Here's how the part is built. I have some questions about the finished solid (model axes, mm). A direction names the side the tool comes from. Give positions to 0.01 mm unless a question says otherwise; leave off trailing zeros. Loops run counter-clockwise (first coordinate to the right, second up) from the corner with the lowest first, then second, coordinate; pieces in that order, holes last. Notation, with made-up numbers: M 22,-19.5 L 64,-19.5 A18 cw 64,-13.5 Z; hole C 82.5,27.25 d9. An arc over 180 degrees is marked long. Answer as CSV lines item,"result". Start each with the question number.
Item 1: I want a section at A-A on y = 10. List the corners of the cut face in (x, z) for me, plus the area to 3 significant figures.
Item 2: If I drill on line 1 along Z through (x, y) = (-7.5, 10); line 2 along X through (y, z) = (11, 10); line 3 along Z through (x, y) = (2, 11), over which ranges is the centre line in solid material (lowest first)? Write a range as from..to.
Item 3: I want a section at B-B on z = 4.5. List the corners of the cut face in (x, y) for me.
Item 4: If we mould it in two halves opening along Y, with no side actions, what happens to faces 1 (the cylindrical face through (5.65, 3.52, -22.27)), 2 (the cylindrical face through (-7.062, 11.341, 8.694)), 3 (the flat face through (5.33, 2, 36.78)), 4 (the flat face through (-4, 0, 5))? For each: released by +Y, released by -Y, zero draft, split by the parting line, or undercut.
Item 5: I want a section at C-C on z = 34.5. List the corners of the cut face in (x, y) for me, plus the area to 3 significant figures.
Item 6: For faces 5 (the cylindrical face through (15.357, 11.341, 8.694)), 6 (the cylindrical face through (4.367, 3.521, 32.966)), 7 (the flat face through (-8.852, 10, 8)), 8 (the flat face through (17.148, 10, 8)), 9 (the cylindrical face through (4.214, 1.014, -28.538)), which set-ups out of +Z, -Z, +X, -X, +Y, -Y let a thin tool reach every point of the face, with its end or its side?
Item 7: I want a section at D-D on x = 32. List the corners of the cut face in (y, z) for me.
Item 8: Will these pins go through, and if not, where does the flat tip stop? P1, Ø8, axis at y = 12, z = 10.5, coming from the -X side; P2, Ø16, axis at x = 4.15, z = 5.46, coming from the +Y side; P3, Ø6, axis at x = -18, z = -15, coming from the +Y side; P4, Ø7, axis at y = 10, z = 5.46, coming from the +X side.
from build123d import *

# Parameters (mm, degrees)
SKETCH1_R           = 40
BOSS_EXTRUDE1_DEPTH = 5
SKETCH2_R           = 5
CUT_EXTRUDE1_DEPTH  = 15
SKETCH3_R           = 5
CUT_EXTRUDE2_DEPTH  = 3
SKETCH5_R           = 1.5
CUT_EXTRUDE3_DEPTH  = 33
BOSS_EXTRUDE2_START = 10
SKETCH6_R           = 10
SKETCH6_R_2         = 5
BOSS_EXTRUDE2_DEPTH = 10
SKETCH10_R          = 2.25
CUT_EXTRUDE4_DEPTH  = 45
BOSS_EXTRUDE3_START = 8
SKETCH11_R          = 3.5
SKETCH11_R_2        = 2.25
BOSS_EXTRUDE3_DEPTH = 8


with BuildPart() as part:
    # Sketch1 → Boss-Extrude1 (new body)
    with BuildSketch(Plane(origin=(0, 0, 0), x_dir=(1, 0, 0), z_dir=(0, 1, 0))):
        with Locations(Location((4.147627533, -5.460766911, 0), (0, 0, 270))):
            Circle(SKETCH1_R)
    extrude(amount=BOSS_EXTRUDE1_DEPTH)

    # Sketch2 → Cut-Extrude1 (cut)
    with BuildSketch(Plane(origin=(0, 5, 0), x_dir=(1, 0, 0), z_dir=(0, 1, 0))):
        with Locations(Location((4.147627533, -5.460766911, 0), (0, 0, 270))):
            Circle(SKETCH2_R)
    extrude(amount=-CUT_EXTRUDE1_DEPTH, mode=Mode.SUBTRACT)

    # Sketch3 → Cut-Extrude2 (cut)
    with BuildSketch(Plane(origin=(0, 5, 0), x_dir=(1, 0, 0), z_dir=(0, 1, 0))):
        with Locations(Location((4.147627533, 27.039233089, 0), (0, 0, 270))):
            Circle(SKETCH3_R)
        with Locations(Location((4.147627533, -37.960766911, 0), (0, 0, 270))):
            Circle(SKETCH3_R)
    extrude(amount=-CUT_EXTRUDE2_DEPTH, mode=Mode.SUBTRACT)

    # Sketch5 → Cut-Extrude3 (cut)
    with BuildSketch(Plane(origin=(0, 2, 0), x_dir=(1, 0, 0), z_dir=(0, 1, 0))):
        with Locations(Location((4.147627533, -37.960766911, 0), (0, 0, 270))):
            Circle(SKETCH5_R)
        with Locations(Location((4.147627533, 27.039233089, 0), (0, 0, 270))):
            Circle(SKETCH5_R)
    extrude(amount=-CUT_EXTRUDE3_DEPTH, mode=Mode.SUBTRACT)

    # Sketch6 → Boss-Extrude2 (add)
    with BuildSketch(Plane(origin=(0, 5, 0), x_dir=(1, 0, 0), z_dir=(0, 1, 0)).offset(BOSS_EXTRUDE2_START)):
        with Locations(Location((4.147627533, -5.460766911, 0), (0, 0, 270))):
            Circle(SKETCH6_R)
        with Locations(Location((4.147627533, -5.460766911, 0), (0, 0, 270))):
            Circle(SKETCH6_R_2, mode=Mode.SUBTRACT)
    extrude(amount=-BOSS_EXTRUDE2_DEPTH)

    # Sketch10 → Cut-Extrude4 (cut, symmetric)
    with BuildSketch(Plane(origin=(4.147627533, 0, 5.460766911), x_dir=(0, 0, -1), z_dir=(1, 0, 0))):
        with Locations((0, 10)):
            Circle(SKETCH10_R)
    extrude(amount=CUT_EXTRUDE4_DEPTH, both=True, mode=Mode.SUBTRACT)

    # Sketch11 → Boss-Extrude3 (add)
    with BuildSketch(Plane(origin=(9.147627533, 0, 5.460766911), x_dir=(0, 0, -1), z_dir=(1, 0, 0)).offset(BOSS_EXTRUDE3_START)):
        with Locations(Location((0, 10, 0), (0, 0, 180))):
            Circle(SKETCH11_R)
        with Locations((0, 10)):
            Circle(SKETCH11_R_2, mode=Mode.SUBTRACT)
    boss_extrude3 = extrude(amount=-BOSS_EXTRUDE3_DEPTH)

    # Mirror1: Boss-Extrude3 across plane
    add(boss_extrude3.mirror(Plane(origin=(4.147627533, 0, 5.460766911), x_dir=(0, 0, 1), z_dir=(1, 0, 0))))


solid = part.part
Result:
1,outline,"M -8.85,1.96 L -5.22,1.96 A10 ccw 13.52,1.96 L 17.15,1.96 L 17.15,3.21 L 8.61,3.21 A5 cw -0.32,3.21 L -8.85,3.21 Z; M -8.85,7.71 L -0.32,7.71 A5 cw 8.61,7.71 L 17.15,7.71 L 17.15,8.96 L 13.52,8.96 A10 ccw -5.22,8.96 L -8.85,8.96 Z"
1,area,"207 mm^2"
2,line 1,"1.96..3.21, 7.71..8.96"
2,line 2,"-4.76..2.05, 6.24..13.06"
2,line 3,"-4.31..0.95, 9.98..15.23"
3,outline,"M -35.84,0 L -0.76,0 L -0.76,7.97 L -8.85,7.97 L -8.85,6.63 L -5.81,6.63 L -5.81,5 L -35.84,5 Z; M -8.85,12.03 L -0.76,12.03 L -0.76,15 L -5.81,15 L -5.81,13.37 L -8.85,13.37 Z; M 9.05,0 L 44.14,0 L 44.14,5 L 14.1,5 L 14.1,6.63 L 17.15,6.63 L 17.15,7.97 L 9.05,7.97 Z; M 9.05,12.03 L 17.15,12.03 L 17.15,13.37 L 14.1,13.37 L 14.1,15 L 9.05,15 Z"
4,face 1,"zero draft"
4,face 2,"undercut"
4,face 3,"released by +Y"
4,face 4,"released by -Y"
5,outline,"M -23.36,0 L 31.66,0 L 31.66,5 L 7.76,5 L 7.76,2 L 0.54,2 L 0.54,5 L -23.36,5 Z"
5,area,"253 mm^2"
6,face 5,"+X"
6,face 6,"+Y"
6,face 7,"+Z, -Z, -X, +Y"
6,face 8,"+Z, -Z, +X, +Y"
6,face 9,"+Y, -Y"
7,outline,"M 0,-23.25 L 5,-23.25 L 5,34.17 L 0,34.17 Z"
8,P1,"x = -8.85"
8,P2,"y = 15"
8,P3,"y = 5"
8,P4,"x = 17.15"
